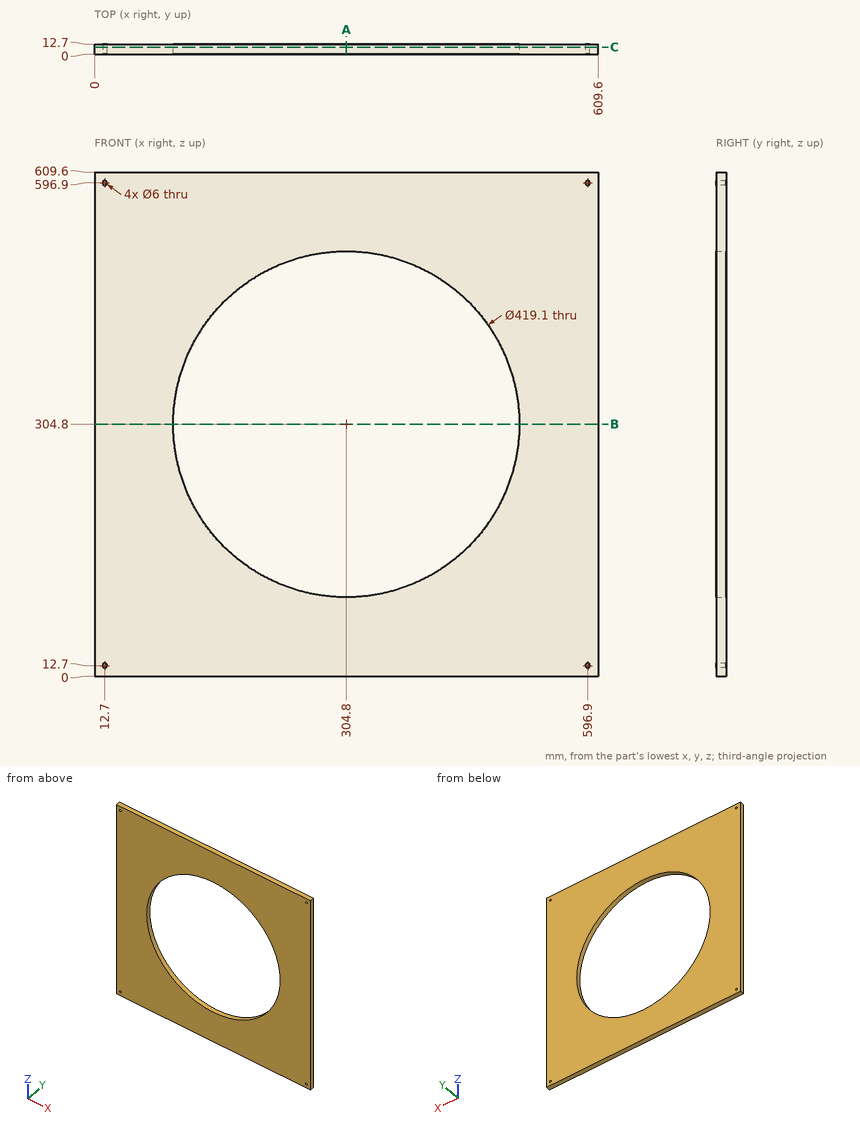
Input: dimensioned drawing with shaded views. Units: mm. Origin: part minimum x, y, z. Round coordinates to 2 decimals unless told otherwise and drop trailing zeros. Loops run counter-clockwise (first coordinate to the right, second up) from the corner with the lowest first, then second, coordinate; pieces in that order, holes last. Notation, with made-up numbers: (14.25, 82) -> (64.25, 82) arc R14 ccw to (64.25, 109) -> close; hole circle Ø5 at (22, 81). An arc over 180 degrees is marked (long way). One line per item, written item: value.
(1) Section C-C (y = 9). Return the cut outline in (x, z), plus the area to 3 significant figures.
Geometry check:
outline: (0, 0) -> (609.6, 0) -> (609.6, 609.6) -> (0, 609.6) -> close; hole circle Ø6 at (12.7, 12.7); hole circle Ø6 at (12.7, 596.9); hole circle Ø419.1 at (304.8, 304.8); hole circle Ø6 at (596.9, 12.7); hole circle Ø6 at (596.9, 596.9)
area: 234,000 mm2
(2) Material intervals for line 1 (Z direction, x = 12.7, y = 7.25); line 2 (Z direction, x = 305, y = 2); line 3 (Z direction, x = 154, y = 2.25), sorted ascending. Write a range as [from, to].
Geometry check:
line 1: [0, 9.7], [15.7, 593.9], [599.9, 609.6]
line 2: [0, 95.25], [514.35, 609.6]
line 3: [0, 159.3], [450.3, 609.6]
(3) Section B-B (z = 304.8). Return the cut outline in (x, y).
Geometry check:
outline: (0, 0) -> (95.25, 0) -> (95.25, 12.7) -> (0, 12.7) -> close; (514.35, 0) -> (609.6, 0) -> (609.6, 12.7) -> (514.35, 12.7) -> close
(4) Pin query (flat end, axial travel): pin 1 (8 mm diameter, centred on x = 12.7, z = 596.9, fed in from +Y); pin 2 (5 mm diameter, centred on x = 596.9, z = 12.7, fed in from +Y). Return the tip coordinate at first contact, or that it passes through.
Geometry check:
pin 1: y = 12.7
pin 2: through
(5) Section A-A (x = 304.8). Return the cut outline in (y, z), plus the area to 3 significant figures.
Geometry check:
outline: (0, 0) -> (12.7, 0) -> (12.7, 95.25) -> (0, 95.25) -> close; (0, 514.35) -> (12.7, 514.35) -> (12.7, 609.6) -> (0, 609.6) -> close
area: 2,420 mm2
